```python
from build123d import *

# Parameters (mm, degrees)
ESQUISSE1_W             = 1000
ESQUISSE1_H             = 1600
ESQUISSE1_R             = 50
ESQUISSE1_W_2           = 600
ESQUISSE1_H_2           = 1200
ESQUISSE1_R_2           = 100
ESQUISSE1_R_3           = 200
BOSS_EXTRU_1_DEPTH      = 250
ESQUISSE3_R             = 200
ENL_V_MAT_EXTRU_1_DEPTH = 150
CONG_1_R                = 120


with BuildPart() as part:
    # Esquisse1 → Boss.-Extru.1 (new body)
    # profile 1 of 3: a face of its own
    with BuildSketch(Plane.XY):
        with Locations((500, 800)):
            Rectangle(ESQUISSE1_W, ESQUISSE1_H)
        with Locations((880, 1480)):
            Circle(ESQUISSE1_R, mode=Mode.SUBTRACT)
        with Locations((120, 1480)):
            Circle(ESQUISSE1_R, mode=Mode.SUBTRACT)
        with Locations((880, 120)):
            Circle(ESQUISSE1_R, mode=Mode.SUBTRACT)
        with Locations((120, 120)):
            Circle(ESQUISSE1_R, mode=Mode.SUBTRACT)
        with Locations((500, 800)):
            Rectangle(ESQUISSE1_W_2, ESQUISSE1_H_2, mode=Mode.SUBTRACT)
    # profile 2 of 3: a face of its own
    with BuildSketch(Plane.XY):
        with Locations((500, 800)):
            Rectangle(ESQUISSE1_W_2, ESQUISSE1_H_2)
        with Locations((620, 1220)):
            Circle(ESQUISSE1_R_2, mode=Mode.SUBTRACT)
        with Locations((380, 380)):
            Circle(ESQUISSE1_R_2, mode=Mode.SUBTRACT)
        with Locations((500, 800)):
            Circle(ESQUISSE1_R_3, mode=Mode.SUBTRACT)
    # profile 3 of 3: a face of its own
    with BuildSketch(Plane.XY):
        with Locations((500, 800)):
            Circle(ESQUISSE1_R_3)
        with Locations((500, 800)):
            Circle(ESQUISSE1_R_2, mode=Mode.SUBTRACT)
    extrude(amount=BOSS_EXTRU_1_DEPTH)

    # Esquisse3 → Enlèv. mat.-Extru.1 (cut)
    with BuildSketch(Plane.XY.offset(250)):
        with BuildLine():
            Line((240, 1400), (760, 1400))
            ThreePointArc((760, 1400), (788.284271247, 1388.284271247), (800, 1360))
            Line((800, 1360), (800, 240))
            ThreePointArc((800, 240), (788.284271247, 211.715728753), (760, 200))
            Line((760, 200), (240, 200))
            ThreePointArc((240, 200), (211.715728753, 211.715728753), (200, 240))
            Line((200, 240), (200, 1360))
            ThreePointArc((200, 1360), (211.715728753, 1388.284271247), (240, 1400))
        make_face()
        with Locations((500, 800)):
            Circle(ESQUISSE3_R, mode=Mode.SUBTRACT)
    extrude(amount=-ENL_V_MAT_EXTRU_1_DEPTH, mode=Mode.SUBTRACT)

    # Congé1
    cong_1_edges = [part.edges().sort_by_distance(p)[0] for p in [
        (0, 0, 125),
        (0, 1600, 125),
        (1000, 1600, 125),
        (1000, 0, 125),
    ]]
    fillet(cong_1_edges, radius=CONG_1_R)


solid = part.part
```
Check sheet for the modelled part. Datum: model origin and axes. Units: mm. A direction names the side the tool comes from. Coordinates: 2 decimals unless noted, no trailing zeros. Order: outer loops, then holes, each group sorted by start corner. A loop starts at its lowest first (then second) coordinate and runs counter-clockwise, first axis right, second up. Notation, with made-up numbers: (-2, 32) -> (52, 32) arc R6 ccw to (52, 36) -> close; hole circle Ø2 at (69.25, -9.75). An arc over 180 degrees is marked (long way). Write item = value, one per line. Start each with the question number.
1) Go/stop test with flat-tipped pins: P1, Ø3, axis at x = 279.5, y = 1317.5, coming from the -Z side; P2, Ø8, axis at x = 411.5, y = 1048, coming from the +Z side. Record where each tip stops, or that it passes through.
2) Mould release check, pull along X, two halves, no side actions. Record for faces 3 (the cylindrical face through (34.219, 36.085, 126.75)), 4 (the cylindrical face through (927.69, 135.02, 123.25)), 5 (the flat face through (826, 811, 250)): +X half, -X half, draft (parallel to the pull), parting line (faces both ways), or undercut.
3) Cross-section at D-D (x = 442.5). Enter the section's corners in (y, z).
4) Cross-section at B-B (y = 800). Enter the section's corners in (x, z), then the cut area to 3 significant figures.
5) Access from +Z, -Z, +X, -X, +Y, -Y to the whole of each face (thin tool, end or side, straight path). Record for faces 1 (the cylindrical face through (34.219, 1563.915, 126.75)), 2 (the flat face through (800, 808, 176)).
6) Cross-section at A-A (z = 210.5). Enter the section's corners in (x, y), then the cut area to 3 significant figures.
7) Material ranges on L1, parallel to Y at x = 120, z = 197; L2, parallel to X at y = 1485.5, z = 88; L3, parallel to X at y = 462.5, z = 185.5, recorded low to high.
8) Cross-section at C-C (x = 620). Enter the section's corners in (y, z), then the cut area to 3 significant figures.
Ans:
q1.P1 = 0
q1.P2 = 100
q2.face_3 = -X half
q2.face_4 = undercut
q2.face_5 = draft
q3.outline = (0, 0) -> (301.94, 0) -> (301.94, 100) -> (200, 100) -> (200, 250) -> (0, 250) -> close; (458.06, 0) -> (718.18, 0) -> (718.18, 250) -> (608.44, 250) -> (608.44, 100) -> (458.06, 100) -> close; (881.82, 0) -> (1600, 0) -> (1600, 250) -> (1400, 250) -> (1400, 100) -> (991.56, 100) -> (991.56, 250) -> (881.82, 250) -> close
q4.outline = (0, 0) -> (400, 0) -> (400, 250) -> (300, 250) -> (300, 100) -> (200, 100) -> (200, 250) -> (0, 250) -> close; (600, 0) -> (1000, 0) -> (1000, 250) -> (800, 250) -> (800, 100) -> (700, 100) -> (700, 250) -> (600, 250) -> close
q4.area = 170,000 mm²
q5.face_1 = +Z, -Z, -X, +Y
q5.face_2 = +Z
q6.outline = (0, 120) arc R120 ccw to (120, 0) -> (880, 0) arc R120 ccw to (1000, 120) -> (1000, 1480) arc R120 ccw to (880, 1600) -> (120, 1600) arc R120 ccw to (0, 1480) -> close; circle Ø400 at (500, 800); hole circle Ø100 at (120, 120); hole circle Ø100 at (120, 1480); hole (200, 240) arc R40 ccw to (240, 200) -> (760, 200) arc R40 ccw to (800, 240) -> (800, 1360) arc R40 ccw to (760, 1400) -> (240, 1400) arc R40 ccw to (200, 1360) -> close; hole circle Ø200 at (500, 800); hole circle Ø100 at (880, 120); hole circle Ø100 at (880, 1480)
q6.area = 932,000 mm²
q7.L1 = 0 to 70, 170 to 1430, 1530 to 1600
q7.L2 = 0.13 to 70.3, 169.7 to 830.3, 929.7 to 999.87
q7.L3 = 0 to 200, 800 to 1000
q8.outline = (0, 0) -> (1120, 0) -> (1120, 100) -> (960, 100) -> (960, 250) -> (640, 250) -> (640, 100) -> (200, 100) -> (200, 250) -> (0, 250) -> close; (1320, 0) -> (1600, 0) -> (1600, 250) -> (1400, 250) -> (1400, 100) -> (1320, 100) -> close
q8.area = 248,000 mm²
